For this review, take the finished solid that the model builds, in its own axes (mm). A direction names the side the tool comes from. Round coordinates to 2 decimals unless told otherwise and drop trailing zeros. Loops run counter-clockwise (first coordinate to the right, second up) from the corner with the lowest first, then second, coordinate; pieces in that order, holes last.
1) Wall thickness on L1, parallel to X at y = 2.75, z = -0.5; L2, parallel to Y at x = 16.75, z = 0 (3 decimals); L3, parallel to Y at x = 16.25, z = -0.75: over which ranges is each line inside the solid? List them lowest first.
2) Tool access review of faces 1 (the flat face through (2.958, 2.028, 3.448)), 2 (the cylindrical face through (16.476, 0.082, 1.873)): name each direction out of +Z, -Z, +X, -X, +Y, -Y from which nothing blocks a thin tool from reaching the whole face with its end or side.
3) Take a section at A-A (x = 10.5). State the section outline as (y, z) points (3 decimals).
4) Insertion check: pin 1 (1.5 mm diameter, centred on x = 10.5, y = -2, fed in from +Z); pin 2 (4 mm diameter, centred on x = 23.5, z = 2, fed in from -Y) (3 decimals). Each pin has a flat end and moves straight along its axis. Give the tip position at first contact, or say it passes through.
```python
from build123d import *

# Parameters (mm, degrees)
Y_KSEKLIK_EKSTR_ZYON1_DEPTH = 6
IZIM2_R                     = 1.875
Y_KSEKLIK_EKSTR_ZYON2_DEPTH = 21.25
IZIM3_OUTSIDE_W             = 51.852
IZIM3_OUTSIDE_H             = 50.614
IZIM3_OUTSIDE_R             = 4
KES_EKSTR_ZYON1_DEPTH       = 10
KES_EKSTR_ZYON1_DRAFT       = -60
IZIM4_OUTSIDE_W             = 51.852
IZIM4_OUTSIDE_H             = 50.614
IZIM4_OUTSIDE_R             = 4
KES_EKSTR_ZYON2_DEPTH       = 10
KES_EKSTR_ZYON2_DRAFT       = -60


with BuildPart() as part:
    # Çizim1 → Yükseklik-Ekstrüzyon1 (new body)
    with BuildSketch(Plane(origin=(0, 0, 0), x_dir=(0, 0, -1), z_dir=(1, 0, 0))):
        Polygon((4.618802154, 0), (2.309401077, 4), (-2.309401077, 4), (-4.618802154, 0), (-2.309401077, -4), (2.309401077, -4), align=None)
    extrude(amount=Y_KSEKLIK_EKSTR_ZYON1_DEPTH)

    # Çizim2 → Yükseklik-Ekstrüzyon2 (add)
    with BuildSketch(Plane(origin=(6, 0, 0), x_dir=(0, 0, -1), z_dir=(1, 0, 0))):
        Circle(IZIM2_R)
    extrude(amount=Y_KSEKLIK_EKSTR_ZYON2_DEPTH)


with BuildPart() as kes_ekstr_zyon1_tool:
    # Çizim3 outside → Kes-Ekstrüzyon1 (with draft: the straight prism first)
    with BuildSketch(Plane(origin=(6, 0, 0), x_dir=(0, 0, -1), z_dir=(1, 0, 0))):
        Rectangle(IZIM3_OUTSIDE_W, IZIM3_OUTSIDE_H)
        Circle(IZIM3_OUTSIDE_R, mode=Mode.SUBTRACT)
    extrude(amount=-KES_EKSTR_ZYON1_DEPTH)
    # Kes-Ekstrüzyon1: the draft: its side faces are tilted about the plane it starts from
    kes_ekstr_zyon1_sides = [kes_ekstr_zyon1_tool.faces().sort_by_distance(p)[0] for p in [
        (1, -25.307, 0),
        (1, 0, -25.926),
        (1, 25.307, 0),
        (1, 0, 25.926),
        (1, 0, 4),
    ]]
    draft(kes_ekstr_zyon1_sides, Plane(origin=(6, 0, 0), x_dir=(0, 0, -1), z_dir=(1, 0, 0)), KES_EKSTR_ZYON1_DRAFT)


with BuildPart() as part_1:
    add(part.part)

    # Kes-Ekstrüzyon1: cut by kes_ekstr_zyon1_tool
    add(kes_ekstr_zyon1_tool.part, mode=Mode.SUBTRACT)


with BuildPart() as kes_ekstr_zyon2_tool:
    # Çizim4 outside → Kes-Ekstrüzyon2 (with draft: the straight prism first)
    with BuildSketch(Plane.ZY):
        Rectangle(IZIM4_OUTSIDE_W, IZIM4_OUTSIDE_H)
        Circle(IZIM4_OUTSIDE_R, mode=Mode.SUBTRACT)
    extrude(amount=-KES_EKSTR_ZYON2_DEPTH)
    # Kes-Ekstrüzyon2: the draft: its side faces are tilted about the plane it starts from
    kes_ekstr_zyon2_sides = [kes_ekstr_zyon2_tool.faces().sort_by_distance(p)[0] for p in [
        (5, -25.307, 0),
        (5, 0, 25.926),
        (5, 25.307, 0),
        (5, 0, -25.926),
        (5, 0, -4),
    ]]
    draft(kes_ekstr_zyon2_sides, Plane.ZY, KES_EKSTR_ZYON2_DRAFT)


with BuildPart() as part_2:
    add(part_1.part)

    # Kes-Ekstrüzyon2: cut by kes_ekstr_zyon2_tool
    add(kes_ekstr_zyon2_tool.part, mode=Mode.SUBTRACT)


solid = part_2.part
```
Response:
1. L1: x = 0 to 6
1. L2: y = -1.875 to 1.875
1. L3: y = -1.72 to 1.72
2. face 1: +Z, +X, -X, +Y
2. face 2: +X
3. outline: circle Ø3.75 at (0, 0)
4. pin 1: stops at z = 1.4
4. pin 2: stops at y = -1.875
